Part print with two shaded views. Sizes in mm from the minimum x, y, z corner. A direction names the side the tool comes from. Give positions to 0.01 mm unless a question says otherwise; leave off trailing zeros. Write each loop counter-clockwise with the first axis right and the second up, starting at its lowest first coordinate (ties: lowest second). Pieces come first, ordered by that corner, then holes. Notation, with made-up numbers: (-8.5, -27) -> (3.5, -27) arc R12 ccw to (3.5, -8) -> close; hole circle Ø2 at (85, 65). An arc over 180 degrees is marked (long way). Use one line per item in the form item = value. Start each with the question number.
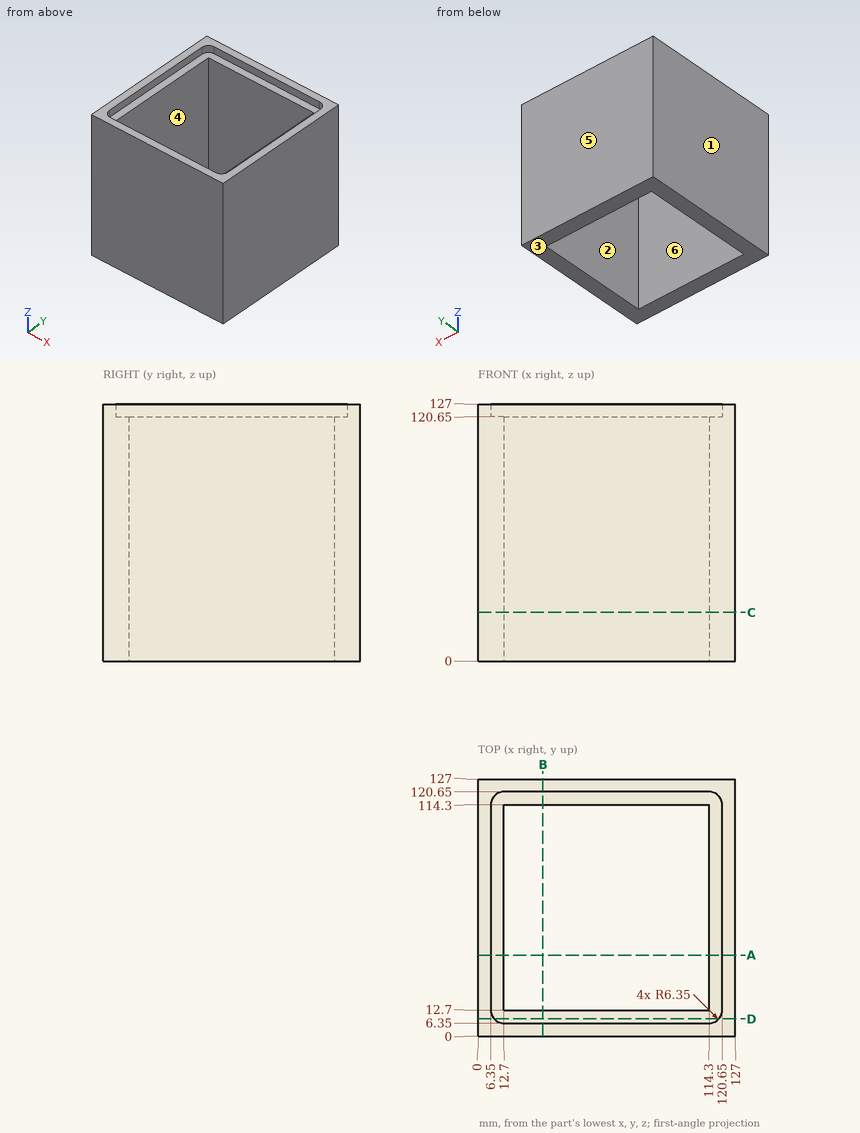
1) 3-axis set-ups, long thin cutter, end or side, ignore diameter. For the marked faces 5 and 6: which of +Z, -Z, +X, -X, +Y, -Y reach the whole face in a straight line?
2) Wall check: line 1 along X through (y, z) = (64.5, 20.5); line 2 along Z through (x, y) = (13, 7). Give the ranges that are in metal, low to high. Write a range as from..to.
3) Cut at C-C (z = 24). Give the cut face in (x, y), and give its area (3 significant figures).
4) Two-plate mould, pull along X, no slides. Class the marked faces 1, 2, 3 and 4: released by +X, released by -X, zero draft, split by the parting line, or undercut.
5) Cut at D-D (y = 8.5). Give the cut face in (x, z), and give its area (3 significant figures).
6) Cut at A-A (y = 40). Give the cut face in (x, z), and give its area (3 significant figures).
Final values:
q1.face_5 = +Z, -Z, +X, -X, +Y
q1.face_6 = +Z, -Z
q2.line_1 = 0..12.7, 114.3..127
q2.line_2 = 0..120.65
q3.outline = (0, 0) -> (127, 0) -> (127, 127) -> (0, 127) -> close; hole (12.7, 12.7) -> (114.3, 12.7) -> (114.3, 114.3) -> (12.7, 114.3) -> close
q3.area = 5,810 mm^2
q4.face_1 = released by -X
q4.face_2 = undercut
q4.face_3 = zero draft
q4.face_4 = undercut
q5.outline = (0, 0) -> (127, 0) -> (127, 127) -> (119.06, 127) -> (119.06, 120.65) -> (7.94, 120.65) -> (7.94, 127) -> (0, 127) -> close
q5.area = 15,400 mm^2
q6.outline = (0, 0) -> (12.7, 0) -> (12.7, 120.65) -> (6.35, 120.65) -> (6.35, 127) -> (0, 127) -> close; (114.3, 0) -> (127, 0) -> (127, 127) -> (120.65, 127) -> (120.65, 120.65) -> (114.3, 120.65) -> close
q6.area = 3,150 mm^2
